Part model, mm, in its own coordinate system. A direction names the side the tool comes from. Round coordinates to 2 decimals unless told otherwise and drop trailing zeros. Loops run counter-clockwise (first coordinate to the right, second up) from the corner with the lowest first, then second, coordinate; pieces in that order, holes last.
(1) Cut at B-B on x = -49.5. List the corners of the cut face in (y, z), then the cut area to 3 significant figures.
(2) Cut at C-C on z = 4. List the corners of the cut face in (x, y), then the cut area to 3 significant figures.
(3) Probe probe 1 along Y at (x, z) = (-4, 3.2); probe 2 along Z at (x, y) = (-67.5, 35); probe 3 along Y at (x, z) = (-35.5, 0.65). List the from-to ranges inside material, lowest first.
(4) Cut at A-A on y = 4.5. List the corners of the cut face in (x, z), then the cut area to 3 significant figures.
(5) Tool access for faces 4 (the face through (-31, 42, 5)), 5 (the face through (-14.978, 40.849, 0.986)): list every direction of +Z, -Z, +X, -X, +Y, -Y with a clear straight run to the whole face (end or side of a thin tool).
(6) Mould opens along Y. For faces 1 (the face through (-48, 64, 1)), 2 (the face through (-12, 35, 0)), 3 (the face through (1.5, 82.4, 2.5)) say: +Y half, -Y half, draft (parallel to the pull), parting line (faces both ways), or undercut.
(7) Flat gauge pins, fed straight in: pin 1 (2 mm diameter, centred on x = -25.5, z = 3.5, fed in from -Y); pin 2 (1 mm diameter, centred on y = 75.5, z = 4.5, fed in from +X); pin 3 (2 mm diameter, centred on x = -67.5, z = 1, fed in from -Y); pin 4 (3.5 mm diameter, centred on x = -76.34, y = 37.05, fed in from +Z). Where does each tip first touch, or does it go through?
Autodesk Inventor part; units mm, degrees
ref_plane "YZ Plane" through (0, 0, 0) normal (1, 0, 0) x (0, 1, 0)
ref_plane "XZ Plane" through (0, 0, 0) normal (0, 1, 0) x (-1, 0, 0)
ref_plane "XY Plane" through (0, 0, 0) normal (0, 0, 1) x (1, 0, 0)
sketch "Sketch1" plane through (0, 0, 0) normal (0, 0, 1) x (1, 0, 0)
  circle A0 centre (0, 0) radius 75 construction
  arc A1 (-78.5195, 32.5529) -> (0, 0) centre (-15.5934, 73.3611) ccw
  line L0 (-15.5934, 73.3611) -> (-78.5195, 32.5529) construction
  line L1 (-15.5934, 73.3611) -> (0, 0) construction
  line L2 (0, 0) -> (64.9519, 37.5) construction
  arc A2 (6.6958, 84.7359) -> (0, 0) centre (64.9519, 37.5) ccw
  line L3 (64.9519, 37.5) -> (6.6958, 84.7359) construction
  line L4 (64.9519, 37.5) -> (0, 0) construction
  line L5 (0, 0) -> (0, 75) construction
  circle A3 centre (0, 0) radius 85 construction
  arc A4 (6.6958, 84.7359) -> (-78.5195, 32.5529) centre (0, 0) ccw
  arc A5 (-74.153, 41.5492) -> (-78.5195, 32.5529) centre (-76.3362, 37.0511) ccw
  line L6 (-76.3362, 37.0511) -> (-78.5195, 32.5529) construction
  line L7 (-76.3362, 37.0511) -> (-74.153, 41.5492) construction
  point P0 (0, 0)
  dimension "d1" = 72
  dimension "d4" = 60
  dimension "d21" = 170
  dimension "d39" = 5
  dimension "d40" = 180
extrude "Extrusion1" add sketch "Sketch1" along normal blind 5
sketch "Sketch3" plane through (0, 0, 5) normal (0, 0, 1) x (1, 0, 0)
  circle A0 centre (0, 0) radius 80 construction
  circle A1 centre (64.9519, 37.5) radius 75
  circle A2 centre (64.9519, 37.5) radius 80 construction
  point P0 (0, 0)
  point P1 (-2.8573, 79.949)
  dimension "d25" = 160
  dimension "d26" = 160
hole "Hole2" at (-2.8573, 79.949, 5) direction (0, 0, -1) diameter 5 end through all
sketch "Sketch4" plane through (0, 0, 5) normal (0, 0, 1) x (1, 0, 0)
  circle A0 centre (-2.8573, 79.949) radius 2.5
  arc A1 (-78.5195, 32.5529) -> (0, 0) centre (-15.5934, 73.3611) ccw
  arc A2 (6.6958, 84.7359) -> (1.3808, 77.2959) centre (64.9519, 37.5) ccw
  arc A3 (6.6958, 84.7359) -> (-3.0359, 84.9458) centre (0, 0) ccw
  arc A4 (6.6958, 84.7359) -> (0, 0) centre (64.9519, 37.5) ccw
  arc A5 (6.6958, 84.7359) -> (-78.5195, 32.5529) centre (0, 0) ccw
  circle A6 centre (-2.8573, 79.949) radius 5
extrude "Extrusion2" cut sketch "Sketch4" against normal blind 10 contours A3 A2 A6
sketch "Sketch5" plane through (0, 0, 5) normal (0, 0, 1) x (1, 0, 0)
  arc A0 (1.3808, 77.2959) -> (-3.0359, 84.9458) centre (-2.8573, 79.949) ccw
  arc A1 (-3.0359, 84.9458) -> (-74.153, 41.5492) centre (0, 0) ccw
  arc A2 (-74.153, 41.5492) -> (-78.5195, 32.5529) centre (-76.3362, 37.0511) ccw
  arc A3 (-78.5195, 32.5529) -> (0, 0) centre (-15.5934, 73.3611) ccw
  arc A4 (1.3808, 77.2959) -> (0, 0) centre (64.9519, 37.5) ccw
  circle A5 centre (-2.8573, 79.949) radius 2.5
  point P0 (0, 0)
hole "Hole3" at (-76.3362, 37.0511, 5) direction (0, 0, -1) diameter 4.134 end through all
sketch "Sketch7" plane through (0, 0, 0) normal (0, 0, -1) x (-1, 0, 0)
  circle A0 centre (76.3362, 37.0511) radius 2.067
  arc A1 (3.0359, 84.9458) -> (-1.3808, 77.2959) centre (2.8573, 79.949) ccw
  arc A2 (0, 0) -> (-1.3808, 77.2959) centre (-64.9519, 37.5) ccw
  arc A3 (0, 0) -> (78.5195, 32.5529) centre (15.5934, 73.3611) ccw
  arc A4 (78.5195, 32.5529) -> (74.153, 41.5492) centre (76.3362, 37.0511) ccw
  arc A5 (74.153, 41.5492) -> (3.0359, 84.9458) centre (0, 0) ccw
  circle A6 centre (2.8573, 79.949) radius 2.5
  arc A7 (71.5064, 35.8724) -> (12.5647, 79.0071) centre (0, 0) ccw
  arc A8 (14.8454, 3.3651) -> (70.9945, 30.5742) centre (15.5934, 73.3611) ccw
  arc A9 (10.2017, 10.0786) -> (7.2658, 71.9181) centre (-64.9519, 37.5) ccw
  arc A10 (10.2017, 10.0786) -> (14.8454, 3.3651) centre (14.8988, 8.3648) ccw
  arc A11 (12.5647, 79.0071) -> (7.2658, 71.9181) centre (11.7794, 74.0692) ccw
  arc A12 (70.9945, 30.5742) -> (71.5064, 35.8724) centre (67.0373, 33.6304) ccw
  point P0 (0, 0)
  dimension "d51" = 5
  dimension "d55" = 5
extrude "Extrusion4" cut sketch "Sketch7" against normal blind 2 contours A12 A8 A10 A9 A11 A7
properties part number "blad"
Final values:
1. outline: (6.46, 0) - (12.12, 0) - (12.12, 2) - (62.85, 2) - (62.85, 0) - (69.1, 0) - (69.1, 5) - (6.46, 5) - close
1. area: 212 mm2
2. outline: (-78.52, 32.55) arc R75 ccw to (0, 0) arc R75 cw to (1.38, 77.3) arc R5 ccw to (-3.04, 84.95) arc R85 ccw to (-74.15, 41.55) arc R5 ccw to start; hole circle Ø4.13 at (-76.34, 37.05); hole circle Ø5 at (-2.86, 79.95)
2. area: 4,520 mm2
3. probe 1: y = -0.74 to 7.99, 67.01 to 77.73, 82.17 to 84.91
3. probe 2: z = 2 to 5
3. probe 3: y = 1.05 to 6.25, 71.69 to 77.23
4. outline: (-45.31, 0) - (-28.17, 0) - (-28.17, 2) - (-11.73, 2) - (-11.73, 0) - (-2.4, 0) - (-2.4, 5) - (-45.31, 5) - close
4. area: 182 mm2
5. face 4: +Z, +X, -X, +Y, -Y
5. face 5: -Z
6. face 1: undercut
6. face 2: draft
6. face 3: parting line
7. pin 1: stops at y = -1.11
7. pin 2: stops at x = 0.59
7. pin 3: stops at y = 18.28
7. pin 4: passes through
